Geometry check sheet. Reference: the model listing, model coordinates, mm. A direction names the side the tool comes from. Give positions to 0.01 mm unless a question says otherwise; leave off trailing zeros. Write each loop counter-clockwise with the first axis right and the second up, starting at its lowest first coordinate (ties: lowest second). Pieces come first, ordered by that corner, then holes. Notation, with made-up numbers: (25, 51) - (60, 51) arc R31 ccw to (60, 83) - close; hole circle Ø11 at (-16.75, -24.75). An arc over 180 degrees is marked (long way). Use a Markdown table: item, result.
```python
from build123d import *

# Parameters (mm, degrees)
SKETCH1_R           = 38.1
SKETCH1_R_2         = 33.02
BOSS_EXTRUDE1_DEPTH = 2.921
SKETCH3_R           = 33.02
SKETCH3_R_2         = 6.35
SKETCH3_R_3         = 1.778
BOSS_EXTRUDE2_DEPTH = 1.5875


with BuildPart() as part:
    # Sketch1 → Boss-Extrude1 (new body, symmetric)
    with BuildSketch(Plane.XY):
        Circle(SKETCH1_R)
        Circle(SKETCH1_R_2, mode=Mode.SUBTRACT)
    extrude(amount=BOSS_EXTRUDE1_DEPTH, both=True)

    # Sketch3 → Boss-Extrude2 (add, symmetric)
    with BuildSketch(Plane.XY):
        Circle(SKETCH3_R)
        Circle(SKETCH3_R_2, mode=Mode.SUBTRACT)
        with Locations((0, 9.779)):
            Circle(SKETCH3_R_3, mode=Mode.SUBTRACT)
        with Locations((6.914797213, 6.914797213)):
            Circle(SKETCH3_R_3, mode=Mode.SUBTRACT)
        with Locations((9.779, 0)):
            Circle(SKETCH3_R_3, mode=Mode.SUBTRACT)
        with Locations((6.914797213, -6.914797213)):
            Circle(SKETCH3_R_3, mode=Mode.SUBTRACT)
        with Locations((0, -9.779)):
            Circle(SKETCH3_R_3, mode=Mode.SUBTRACT)
        with Locations((-6.914797213, -6.914797213)):
            Circle(SKETCH3_R_3, mode=Mode.SUBTRACT)
        with Locations((-9.779, 0)):
            Circle(SKETCH3_R_3, mode=Mode.SUBTRACT)
        with Locations((-6.914797213, 6.914797213)):
            Circle(SKETCH3_R_3, mode=Mode.SUBTRACT)
    extrude(amount=BOSS_EXTRUDE2_DEPTH, both=True)


solid = part.part
```
1) Section check C-C on x = -10.5. Record the boundary of the cut face in (y, z).
Working result:
| item | result |
|---|---|
| outline | (-36.62, -2.92) - (-31.31, -2.92) - (-31.31, -1.59) - (-1.63, -1.59) - (-1.63, 1.59) - (-31.31, 1.59) - (-31.31, 2.92) - (-36.62, 2.92) - close; (1.63, -1.59) - (31.31, -1.59) - (31.31, -2.92) - (36.62, -2.92) - (36.62, 2.92) - (31.31, 2.92) - (31.31, 1.59) - (1.63, 1.59) - close |
2) Section check A-A on y = 0. Record the boundary of the cut face in (x, z), then the cut area to 3 significant figures.
Working result:
| item | result |
|---|---|
| outline | (-38.1, -2.92) - (-33.02, -2.92) - (-33.02, -1.59) - (-11.56, -1.59) - (-11.56, 1.59) - (-33.02, 1.59) - (-33.02, 2.92) - (-38.1, 2.92) - close; (-8, -1.59) - (-6.35, -1.59) - (-6.35, 1.59) - (-8, 1.59) - close; (6.35, -1.59) - (8, -1.59) - (8, 1.59) - (6.35, 1.59) - close; (11.56, -1.59) - (33.02, -1.59) - (33.02, -2.92) - (38.1, -2.92) - (38.1, 2.92) - (33.02, 2.92) - (33.02, 1.59) - (11.56, 1.59) - close |
| area | 206 mm² |
3) Depth check by flat-ended pin: P1, Ø2, axis at x = 4, y = -29.5, coming from the +Z side; P2, Ø2, axis at y = -17.5, z = 0.5, coming from the -X side; P3, Ø3, axis at y = -7.5, z = -2, coming from the -X side. Enter the tip coordinate at first touch or a pass-through.
Working result:
| item | result |
|---|---|
| P1 | stops at z = 1.59 |
| P2 | stops at x = -34.34 |
| P3 | stops at x = -37.62 |
4) Mould release check, pull along X, two halves, no side actions. Record for faces 4 (the cylindrical face through (5.604, -5.713, -0.022)), 5 (the flat face through (-11.5, 31.2, -2.921)), 6 (the cylindrical face through (-30.235, -23.183, 0.041)): pulls with the +X half, pulls with the -X half, needs draft (parallel to the pull), parting line crosses it, or undercut.
Working result:
| item | result |
|---|---|
| face 4 | undercut |
| face 5 | needs draft |
| face 6 | parting line crosses it |
5) Set-up check for faces 1 (the flat face through (-11.5, 31.2, 2.921)), 2 (the cylindrical face through (31.5, 9.9, -2.3)), 3 (the cylindrical face through (31.5, 9.9, 2.2)): record each of +Z, -Z, +X, -X, +Y, -Y from which the full face is reachable in a straight line by a thin tool's end or side.
Working result:
| item | result |
|---|---|
| face 1 | +Z, +X, -X, +Y, -Y |
| face 2 | -Z |
| face 3 | +Z |
6) Section check D-D on z = 0.25. Count the separate pieces of the cut face and the enclosed holes in it, then the cut area to 3 significant figures.
Working result:
| item | result |
|---|---|
| separate pieces | 1 |
| enclosed holes | 9 |
| area | 4,350 mm² |
7) Material ranges on L1, parallel to X at y = 0.5, z = -1.65; L2, parallel to Y at x = 1, z = -2.55; L3, parallel to Y at x = 6.5, z = -0.1, recorded low to high. Write a range as from..to.
Working result:
| item | result |
|---|---|
| L1 | x = -38.1..-33.02, 33.02..38.1 |
| L2 | y = -38.09..-33, 33..38.09 |
| L3 | y = -37.54..-8.64, -5.19..5.19, 8.64..37.54 |
